from build123d import *

# Parameters (mm, degrees)
SKETCH1_R           = 2.5
SKETCH1_R_2         = 4
BOSS_EXTRUDE1_DEPTH = 3
BOSS_EXTRUDE2_DEPTH = 26
BOSS_EXTRUDE3_DEPTH = 0.75


with BuildPart() as part:
    # Sketch1 → Boss-Extrude1 (new body)
    with BuildSketch(Plane.XY):
        with BuildLine():
            Line((-44, 18), (-72.807966597, 18))
            ThreePointArc((-72.807966597, 18), (-75, 0), (-72.807966597, -18))
            Line((-72.807966597, -18), (-44, -18))
            Line((-44, -18), (-36, -10))
            Line((-36, -10), (-16, -10))
            Line((-16, -10), (-8, -18))
            Line((-8, -18), (8, -18))
            Line((8, -18), (16, -10))
            Line((16, -10), (36, -10))
            Line((36, -10), (44, -18))
            Line((44, -18), (72.807966597, -18))
            ThreePointArc((72.807966597, -18), (74.449974798, -9.066490645), (75, 0))
            ThreePointArc((75, 0), (74.449974798, 9.066490645), (72.807966597, 18))
            Line((72.807966597, 18), (44, 18))
            Line((44, 18), (36, 10))
            Line((36, 10), (16, 10))
            Line((16, 10), (8, 18))
            Line((8, 18), (-8, 18))
            Line((-8, 18), (-16, 10))
            Line((-16, 10), (-36, 10))
            Line((-36, 10), (-44, 18))
        make_face()
        with Locations((-45, 0)):
            Circle(SKETCH1_R, mode=Mode.SUBTRACT)
        Circle(SKETCH1_R_2, mode=Mode.SUBTRACT)
        with Locations((45, 0)):
            Circle(SKETCH1_R, mode=Mode.SUBTRACT)
    extrude(amount=BOSS_EXTRUDE1_DEPTH)

    # Sketch2 → Boss-Extrude2 (add)
    with BuildSketch(Plane.XY.offset(3)):
        with BuildLine():
            ThreePointArc((69.713700232, 18), (72, 0), (69.713700232, -18))
            Line((69.713700232, -18), (72.807966597, -18))
            ThreePointArc((72.807966597, -18), (75, 0), (72.807966597, 18))
            Line((72.807966597, 18), (69.713700232, 18))
        make_face()
        with BuildLine():
            ThreePointArc((-72.807966597, 18), (-75, 0), (-72.807966597, -18))
            Line((-72.807966597, -18), (-69.713700232, -18))
            ThreePointArc((-69.713700232, -18), (-72, 0), (-69.713700232, 18))
            Line((-69.713700232, 18), (-72.807966597, 18))
        make_face()
    extrude(amount=BOSS_EXTRUDE2_DEPTH)

    # Sketch3 → Boss-Extrude3 (add, symmetric)
    with BuildSketch(Plane(origin=(0, 0, 0), x_dir=(-1, 0, 0), z_dir=(0, -1, 0))):
        Polygon((-72, -3), (-57, -3), (-72, -29), align=None)
        Polygon((72, -29), (72, -3), (57, -3), align=None)
    boss_extrude3 = extrude(amount=BOSS_EXTRUDE3_DEPTH, both=True)

    # Mirror1: Boss-Extrude3 across plane
    add(boss_extrude3.mirror(Plane(origin=(0, 0, 0), x_dir=(0, 0, 1), z_dir=(1, 0, 0))))


solid = part.part
The model under review builds one solid part; all positions refer to its coordinate system, in mm. A direction names the side the tool comes from. Round coordinates to 2 decimals unless told otherwise and drop trailing zeros. Loops run counter-clockwise (first coordinate to the right, second up) from the corner with the lowest first, then second, coordinate; pieces in that order, holes last. Notation, with made-up numbers: (46, -22.5) -> (86, -22.5) arc R13 cw to (86, -5.5) -> close; hole circle Ø5 at (7, 53). An arc over 180 degrees is marked (long way). Return JSON: item names as keys, results as strings.
(1) For pin 1 (5 mm diameter, centred on y = -12, z = 10.5, fed in from -X); pin 2 (4.5 mm diameter, centred on x = -66.5, z = 10, fed in from -Y); pin 3 (2.5 mm diameter, centred on x = -21.5, z = 1, fed in from +Y); pin 4 (1 mm diameter, centred on x = -15.5, z = 4.5, fed in from +Y), all flat-tipped, find the tip position at first contact; note any pin that passes through.
Solved:
{"pin 1": "x = -74.4", "pin 2": "y = -0.75", "pin 3": "y = 10", "pin 4": "through"}
(2) For line 1 (Y direction, x = -45, z = 0.95); line 2 (Y direction, x = 0, z = 0.9); line 3 (X direction, y = 1.5, z = 9.5) (3 decimals), list the stretches that pass through material, from the lowest coordinate up.
Solved:
{"line 1": "-18 to -2.5, 2.5 to 18", "line 2": "-18 to -4, 4 to 18", "line 3": "-74.985 to -71.984, 71.984 to 74.985"}
(3) For faces 1 (the flat face through (-12, 14, 1)), 2 (the flat face through (40, -14, 1)), 3 (the flat face through (-1, 4.3, 0)), 4 (the cylindrical face through (71.41, 9.2, 15.82)), list the 3-axis set-ups (+Z, -Z, +X, -X, +Y, -Y) from which the entire face can be reached by the end or side of a thin tool; tool diameter is ignored.
Solved:
{"face 1": "+Z, -Z, +Y", "face 2": "+Z, -Z, -Y", "face 3": "-Z, +X, -X, +Y, -Y", "face 4": "+Z"}
(4) The part is to be moulded in two halves that separate along Y. For faces 5 (the flat face through (-40, 14, 1)), 6 (the flat face through (0, -18, 1)), 7 (the cylindrical face through (-0.867, -3.905, 1.479)), say which applies: released by +Y, released by -Y, zero draft, split by the parting line, or undercut.
Solved:
{"face 5": "released by +Y", "face 6": "released by -Y", "face 7": "undercut"}
(5) Add section D-D on x = -19. Write out the cut boundary in (y, z), plus the area to 3 significant figures.
Solved:
{"outline": "(-10, 0) -> (10, 0) -> (10, 3) -> (-10, 3) -> close", "area": "60.0 mm2"}
(6) Add section C-C on y = 13.5. Write out the cut boundary in (x, z) (3 decimals).
Solved:
{"outline": "(-73.775, 0) -> (-39.5, 0) -> (-39.5, 3) -> (-70.723, 3) -> (-70.723, 29) -> (-73.775, 29) -> close; (-12.5, 0) -> (12.5, 0) -> (12.5, 3) -> (-12.5, 3) -> close; (39.5, 0) -> (73.775, 0) -> (73.775, 29) -> (70.723, 29) -> (70.723, 3) -> (39.5, 3) -> close"}
(7) Add section A-A on x = 0. Write out the cut boundary in (y, z), plus the area to 3 significant figures.
Solved:
{"outline": "(-18, 0) -> (-4, 0) -> (-4, 3) -> (-18, 3) -> close; (4, 0) -> (18, 0) -> (18, 3) -> (4, 3) -> close", "area": "84.0 mm2"}
(8) Add section B-B on z = 10.5. Write out the cut boundary in (x, y), plus the area to 3 significant figures.
Solved:
{"outline": "(-72.81, -18) -> (-69.71, -18) arc R72 cw to (-72, -0.75) -> (-61.33, -0.75) -> (-61.33, 0.75) -> (-72, 0.75) arc R72 cw to (-69.71, 18) -> (-72.81, 18) arc R75 ccw to start; (61.33, -0.75) -> (72, -0.75) arc R72 cw to (69.71, -18) -> (72.81, -18) arc R75 ccw to (72.81, 18) -> (69.71, 18) arc R72 cw to (72, 0.75) -> (61.33, 0.75) -> close", "area": "250 mm2"}
